Geometry: final body of the model. Coordinates: model frame, mm. A direction names the side the tool comes from. Coordinates: 2 decimals unless noted, no trailing zeros. Order: outer loops, then holes, each group sorted by start corner. A loop starts at its lowest first (then second) coordinate and runs counter-clockwise, first axis right, second up. Notation, with made-up numbers: (-26, 38.5) -> (-17, 38.5) arc R28 ccw to (-17, 63.5) -> close; hole circle Ø4 at (-6, -24). An arc over 180 degrees is marked (long way). Answer in a Markdown table with one row per item. Add a question column.
1) Contact query for a flat-ended pin moving along its axis: P1, Ø16, axis at x = -2, y = 0.5, coming from the +Z side. Output: stop coordinate, or through.
2) Set-up query: faces 5 (the face through (0, 10, 3)), 6 (the face through (0, -15, 2)). Return all of +Z, -Z, +X, -X, +Y, -Y with unobstructed straight access to the full face (end or side cutting, diameter ignored); none if empty.
3) Section query A-A on y = -13. Return the cut outline in (x, z).
4) Section query B-B on z = 2.95. Return the cut outline in (x, y).
5) Pull-direction query (X, two-part tool) for faces 1 (the face through (0, 15, 2)), 2 (the face through (17.02, -13.76, 2.03)), 3 (the face through (17.02, 12.24, 2.03)), 4 (the face through (20, 0, 2)); classes: +X half, -X half, draft (parallel to the pull), parting line (faces both ways), or undercut.
6) Section query C-C on x = -17.5. Return the cut outline in (y, z).
7) Section query D-D on x = 2. Return the cut outline in (y, z).
8) Ray query, line 1 (X direction, y = 13, z = 2.05); line 2 (Y direction, x = -17.5, z = 1.2); line 3 (Y direction, x = 11, z = 3.4). Return the intervals inside material, ascending. Write a range as from..to.
```python
from build123d import *

# Parameters (mm, degrees)
SKETCH1_W           = 40
SKETCH1_H           = 30
BOSS_EXTRUDE1_DEPTH = 4
CUT_EXTRUDE1_START  = 4
SKETCH2_W           = 36
SKETCH2_H           = 20
CUT_EXTRUDE1_DEPTH  = 3
CUT_EXTRUDE2_START  = 4
SKETCH3_R           = 0.9
CUT_EXTRUDE2_DEPTH  = 13


with BuildPart() as part:
    # Sketch1 → Boss-Extrude1 (new body)
    with BuildSketch(Plane.XY):
        Rectangle(SKETCH1_W, SKETCH1_H)
    extrude(amount=BOSS_EXTRUDE1_DEPTH)

    # Sketch2 → Cut-Extrude1 (cut)
    with BuildSketch(Plane.XY.offset(CUT_EXTRUDE1_START)):
        Rectangle(SKETCH2_W, SKETCH2_H)
    extrude(amount=-CUT_EXTRUDE1_DEPTH, mode=Mode.SUBTRACT)

    # Sketch3 → Cut-Extrude2 (cut)
    with BuildSketch(Plane.XY.offset(CUT_EXTRUDE2_START)):
        with Locations(Location((-17.5, 13, 0), (0, 0, 180))):
            Circle(SKETCH3_R)
        with Locations(Location((-17.5, -13, 0), (0, 0, 180))):
            Circle(SKETCH3_R)
        with Locations(Location((17.5, -13, 0), (0, 0, 180))):
            Circle(SKETCH3_R)
        with Locations(Location((17.5, 13, 0), (0, 0, 180))):
            Circle(SKETCH3_R)
    extrude(amount=-CUT_EXTRUDE2_DEPTH, mode=Mode.SUBTRACT)


solid = part.part
```
Result:
| question | item | result |
|---|---|---|
| 1 | P1 | z = 1 |
| 2 | face 5 | +Z |
| 2 | face 6 | +Z, -Z, +X, -X, -Y |
| 3 | outline | (-20, 0) -> (-18.4, 0) -> (-18.4, 4) -> (-20, 4) -> close; (-16.6, 0) -> (16.6, 0) -> (16.6, 4) -> (-16.6, 4) -> close; (18.4, 0) -> (20, 0) -> (20, 4) -> (18.4, 4) -> close |
| 4 | outline | (-20, -15) -> (20, -15) -> (20, 15) -> (-20, 15) -> close; hole circle Ø1.8 at (-17.5, -13); hole circle Ø1.8 at (-17.5, 13); hole (-18, -10) -> (18, -10) -> (18, 10) -> (-18, 10) -> close; hole circle Ø1.8 at (17.5, -13); hole circle Ø1.8 at (17.5, 13) |
| 5 | face 1 | draft |
| 5 | face 2 | undercut |
| 5 | face 3 | undercut |
| 5 | face 4 | +X half |
| 6 | outline | (-15, 0) -> (-13.9, 0) -> (-13.9, 4) -> (-15, 4) -> close; (-12.1, 0) -> (12.1, 0) -> (12.1, 4) -> (10, 4) -> (10, 1) -> (-10, 1) -> (-10, 4) -> (-12.1, 4) -> close; (13.9, 0) -> (15, 0) -> (15, 4) -> (13.9, 4) -> close |
| 7 | outline | (-15, 0) -> (15, 0) -> (15, 4) -> (10, 4) -> (10, 1) -> (-10, 1) -> (-10, 4) -> (-15, 4) -> close |
| 8 | line 1 | -20..-18.4, -16.6..16.6, 18.4..20 |
| 8 | line 2 | -15..-13.9, -12.1..-10, 10..12.1, 13.9..15 |
| 8 | line 3 | -15..-10, 10..15 |
